The model under review builds one solid part; all positions refer to its coordinate system, in mm. Face numbers are marked on the shaded views. A direction names the side the tool comes from. Round coordinates to 2 decimals unless told otherwise and drop trailing zeros. Loops run counter-clockwise (first coordinate to the right, second up) from the corner with the lowest first, then second, coordinate; pieces in that order, holes last. Notation, with made-up numbers: (-12, 63) -> (43, 63) arc R20 cw to (43, 87) -> close; hole circle Ø4 at (-19, 2.25). An arc over 180 degrees is marked (long way). Use CSV: the item, a comma, the result in double quotes. Start each with the question number.
```python
from build123d import *

# Parameters (mm, degrees)
CUT_EXTRUDE3_DEPTH      = 139.585713549
CUT_EXTRUDE3_DEPTH_BACK = 139.585713549
SKETCH3_R               = 3


with BuildPart() as part:
    # Sketch1 → Revolve1 (revolve)
    with BuildSketch(Plane(origin=(0, 0, 0), x_dir=(1, 0, 0), z_dir=(0, 1, 0)), mode=Mode.PRIVATE) as revolve1_sk:
        Polygon((0, 0), (0, 6), (7, 6), (7, 4), (13, 4), (13, 6), (22, 6), (22, 9), (104, 9), (104, 7), (114, 7), (114, 9), (138, 9), (138, 0), align=None)
    revolve(revolve1_sk.sketch.rotate(Axis((0, 0, 0), (1, 0, 0)), 180), axis=Axis((0, 0, 0), (1, 0, 0)))

    # Sketch3 → Cut-Extrude3 (cut, two sides: drawn at the far end of the back side and taken through both)
    with BuildSketch(Plane(origin=(0, 0, 0), x_dir=(1, 0, 0), z_dir=(0, 1, 0)).offset(-CUT_EXTRUDE3_DEPTH_BACK)):
        with Locations(Location((126, 0, 0), (0, 0, 90))):
            Circle(SKETCH3_R)
    extrude(amount=CUT_EXTRUDE3_DEPTH + CUT_EXTRUDE3_DEPTH_BACK, mode=Mode.SUBTRACT)


solid = part.part
```
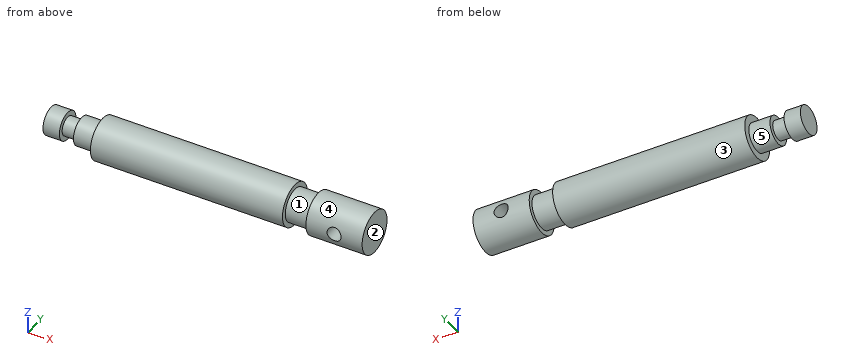
1. Take a section at B-B, the plane y = 0. Give the boundary of the cut face in (x, z), then the cut area to 3 significant figures.
2. Take a section at D-D, the plane x = 126. Give the boundary of the cut face in (y, z).
3. Take a section at C-C, the plane x = 98.5. Give the boundary of the cut face in (y, z).
4. For line 1 along X through (y, z) = (-5, 0); line 2 along X through (y, z) = (0.25, 0); line 3 along X through (y, z) = (5, -6), list the stretches that pass through material, from the lowest coordinate up. Write a range as from..to.
5. The part is to be moulded in two halves that separate along X. For the marked faces 1, 2 and 3, say which applies: pulls with the +X half, pulls with the -X half, needs draft (parallel to the pull), parting line crosses it, or undercut.
6. Take a section at A-A, the plane z = 0. Give the boundary of the cut face in (x, y).
7. Clearance check with flat-ended pins moving along their axes: P1, Ø2, axis at x = 15, z = 0.5, coming from the +Y side; P2, Ø8, axis at x = 45.5, z = 4.5, coming from the -Y side; P3, Ø5, axis at x = 35.5, z = 3, coming from the +Y side. State where each tip first meets the part, or that it passes through.
8. For the marked faces 4 and 5, list the 3-axis set-ups (+Z, -Z, +X, -X, +Y, -Y) from which the entire face can be reached by the end or side of a thin tool; tool diameter is ignored.
Results:
1,outline,"(0, -6) -> (7, -6) -> (7, -4) -> (13, -4) -> (13, -6) -> (22, -6) -> (22, -9) -> (104, -9) -> (104, -7) -> (114, -7) -> (114, -9) -> (138, -9) -> (138, 9) -> (114, 9) -> (114, 7) -> (104, 7) -> (104, 9) -> (22, 9) -> (22, 6) -> (13, 6) -> (13, 4) -> (7, 4) -> (7, 6) -> (0, 6) -> close; hole circle Ø6 at (126, 0)"
1,area,"2,260 mm²"
2,outline,"(-8.49, -3) arc R9 ccw to (8.49, -3) -> close; (-8.49, 3) -> (8.49, 3) arc R9 ccw to start"
3,outline,"circle Ø18 at (0, 0)"
4,line 1,"0..7, 13..123, 129..138"
4,line 2,"0..123, 129..138"
4,line 3,"22..104, 114..138"
5,face 1,"undercut"
5,face 2,"pulls with the +X half"
5,face 3,"needs draft"
6,outline,"(0, -6) -> (7, -6) -> (7, -4) -> (13, -4) -> (13, -6) -> (22, -6) -> (22, -9) -> (104, -9) -> (104, -7) -> (114, -7) -> (114, -9) -> (123, -9) -> (123, 9) -> (114, 9) -> (114, 7) -> (104, 7) -> (104, 9) -> (22, 9) -> (22, 6) -> (13, 6) -> (13, 4) -> (7, 4) -> (7, 6) -> (0, 6) -> close; (129, -9) -> (138, -9) -> (138, 9) -> (129, 9) -> close"
7,P1,"y = 6"
7,P2,"y = -8.99"
7,P3,"y = 8.99"
8,face 4,"+X, -X"
8,face 5,"-X"
